```python
from build123d import *

# Parameters (mm, degrees)
SKETCH1_R           = 2.286
BOSS_EXTRUDE1_DEPTH = 2.54
SKETCH2_R           = 1.905
BOSS_EXTRUDE2_DEPTH = 5.08
CHAMFER1_SIZE       = 2.54


with BuildPart() as part:
    # Sketch1 → Boss-Extrude1 (new body)
    with BuildSketch(Plane.XY):
        with BuildLine():
            Line((22.654726315, 7.62), (25.4, 7.62))
            Line((25.4, 7.62), (25.4, 0))
            Line((25.4, 0), (0, 0))
            Line((0, 0), (0, 7.62))
            Line((0, 7.62), (2.745273685, 7.62))
            ThreePointArc((2.745273685, 7.62), (6.061453031, 8.554701805), (8.401368182, 11.083636364))
            ThreePointArc((8.401368182, 11.083636364), (12.7, 13.716), (16.998631818, 11.083636364))
            ThreePointArc((16.998631818, 11.083636364), (19.338546969, 8.554701805), (22.654726315, 7.62))
        make_face()
        with Locations((3.81, 3.81)):
            Circle(SKETCH1_R, mode=Mode.SUBTRACT)
        with Locations((21.59, 3.81)):
            Circle(SKETCH1_R, mode=Mode.SUBTRACT)
    extrude(amount=BOSS_EXTRUDE1_DEPTH)

    # Sketch2 → Boss-Extrude2 (add)
    with BuildSketch(Plane.XY.offset(2.54)):
        with Locations((12.7, 8.89)):
            Circle(SKETCH2_R)
    extrude(amount=BOSS_EXTRUDE2_DEPTH)

    # Chamfer1
    chamfer1_edges = [part.edges().sort_by_distance(p)[0] for p in [
        (0, 7.62, 1.27),
        (25.4, 7.62, 1.27),
        (25.4, 0, 1.27),
        (0, 0, 1.27),
    ]]
    chamfer(chamfer1_edges, length=CHAMFER1_SIZE)


solid = part.part
```
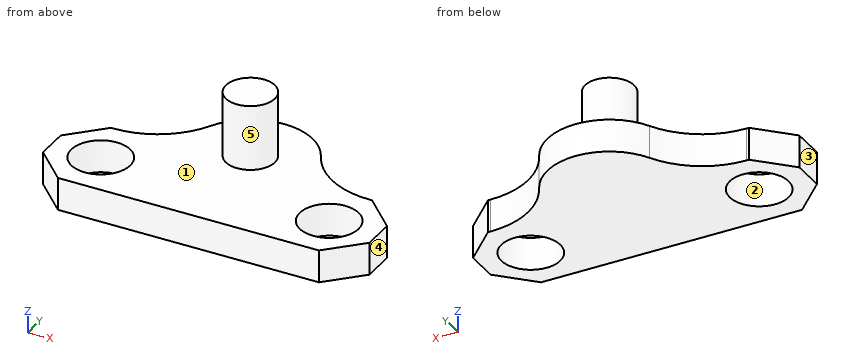
Model file for the job. Use its own axes, mm. Face numbers are marked on the shaded views. A direction names the side the tool comes from. Round coordinates to 2 decimals unless told otherwise and drop trailing zeros. Write each loop counter-clockwise with the first axis right and the second up, starting at its lowest first coordinate (ties: lowest second). Pieces come first, ordered by that corner, then holes. Notation, with made-up numbers: M -24.75,40 L -3.75,40 A33 ccw -3.75,72 Z; hole C 85,38.5 d9. An arc over 180 degrees is marked long. Put each result on its own line as item: value.
Item 1: Cut at B-B (y = 3.81). List the corners of the cut face in (x, z).
Responses:
outline: M 0,0 L 1.52,0 L 1.52,2.54 L 0,2.54 Z; M 6.1,0 L 19.3,0 L 19.3,2.54 L 6.1,2.54 Z; M 23.88,0 L 25.4,0 L 25.4,2.54 L 23.88,2.54 Z
Item 2: Cut at C-C (x = 5.25). List the corners of the cut face in (y, z).
Responses:
outline: M 0,0 L 2.03,0 L 2.03,2.54 L 0,2.54 Z; M 5.59,0 L 8.13,0 L 8.13,2.54 L 5.59,2.54 Z
Item 3: Flat gauge pins, fed straight in: P1, Ø1.5, axis at y = 9.5, z = 6, coming from the -X side (3 decimals); P2, Ø3, axis at y = 8, z = 1.5, coming from the +X side; P3, Ø1.5, axis at x = 17.5, y = 9.5, coming from the +Z side. Where does each tip first touch, or does it go through?
Responses:
P1: x = 10.795
P2: x = 23.98
P3: z = 2.54
Item 4: Mould opens along X. For the marked faces 1, 2 and 3 say: +X half, -X half, draft (parallel to the pull), parting line (faces both ways), or undercut.
Responses:
face 1: draft
face 2: undercut
face 3: -X half
Item 5: Cut at D-D (x = 12.7). List the corners of the cut face in (y, z) (3 decimals).
Responses:
outline: M 0,0 L 13.716,0 L 13.716,2.54 L 10.795,2.54 L 10.795,7.62 L 6.985,7.62 L 6.985,2.54 L 0,2.54 Z
Item 6: Cut at A-A (z = 2.25). List the corners of the cut face in (x, y).
Responses:
outline: M 0,2.54 L 2.54,0 L 22.86,0 L 25.4,2.54 L 25.4,5.08 L 22.86,7.62 L 22.65,7.62 A6.35 cw 17,11.08 A4.83 ccw 8.4,11.08 A6.35 cw 2.75,7.62 L 2.54,7.62 L 0,5.08 Z; hole C 3.81,3.81 d4.57; hole C 21.59,3.81 d4.57
Item 7: Probe L1, parallel to X at y = 2.75, z = 1.25; L2, parallel to X at y = 5.5, z = 2.5; L3, parallel to Z at x = 16, y = 8.25. List the from-to ranges inside material, lowest first. Write a range as from..to.
Responses:
L1: 0..1.78, 5.84..19.56, 23.62..25.4
L2: 0.42..2.27, 5.35..20.05, 23.13..24.98
L3: 0..2.54
Item 8: Tool access for the marked faces 4 and 5: list every direction of +Z, -Z, +X, -X, +Y, -Y with a clear straight run to the whole face (end or side of a thin tool).
Responses:
face 4: +Z, -Z, +X, +Y, -Y
face 5: +Z
